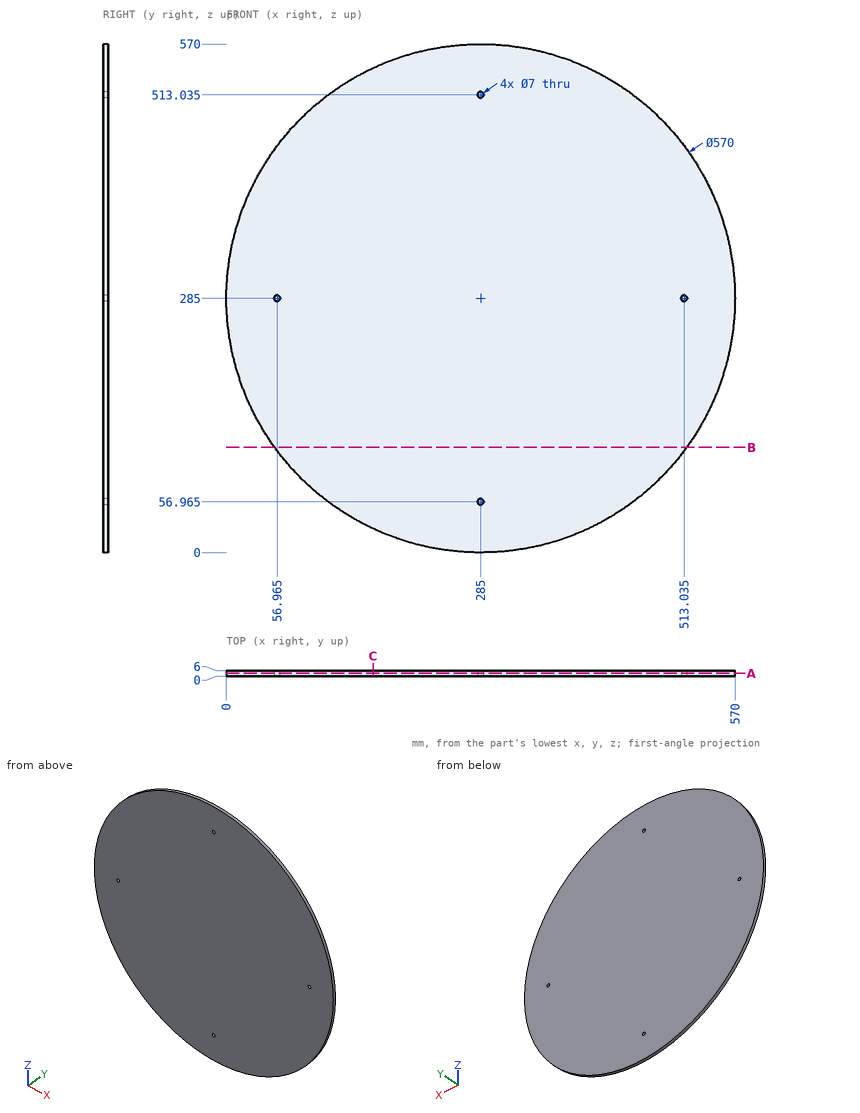
Geometry: see drawing. Coordinates: mm, zero at the bounding-box minimum. Coordinates: 2 decimals unless noted, no trailing zeros. Loops run counter-clockwise (first coordinate to the right, second up) from the corner with the lowest first, then second, coordinate; pieces in that order, holes last. Notation, with made-up numbers: (45.25, 62.25) - (100.25, 62.25) arc R8 ccw to (100.25, 69.25) - close; hole circle Ø6 at (75, 44.25). An arc over 180 degrees is marked (long way). Return JSON: item names as keys, results as strings.
Q1. Contact query for flat-ended pins moving along their axis: P1, Ø1, axis at x = 409, y = 1, coming from the -Z side; P2, Ø1.5, axis at x = 228, y = 1.5, coming from the -Z side. Output: stop coordinate, or through.
Results:
{"P1": "z = 28.15", "P2": "z = 5.61"}
Q2. Material intervals for line 1 along X through (y, z) = (4.6, 285) (3 decimals); line 2 along Z through (x, y) = (510, 0.65), sorted ascending.
Results:
{"line 1": "0 to 53.465, 60.465 to 509.535, 516.535 to 570", "line 2": "110.07 to 283.26, 286.74 to 459.93"}
Q3. Section B-B, the plane z = 118. Return loops of the section in (x, y).
Results:
{"outline": "(54.05, 0) - (515.95, 0) - (515.95, 6) - (54.05, 6) - close"}
Q4. Section A-A, the plane y = 2.95. Return loops of the section in (x, z) (3 decimals).
Results:
{"outline": "circle Ø570 at (285, 285); hole circle Ø7 at (56.965, 285); hole circle Ø7 at (285, 56.965); hole circle Ø7 at (285, 513.035); hole circle Ø7 at (513.035, 285)"}
Q5. Section C-C, the plane x = 164.5. Return loops of the section in (y, z), plus the area to 3 significant figures.
Results:
{"outline": "(0, 26.73) - (6, 26.73) - (6, 543.27) - (0, 543.27) - close", "area": "3,100 mm2"}
